```python
from build123d import *

# Parameters (mm, degrees)
SKETCH_1_W      = 54
SKETCH_1_H      = 35
EXTRUDE_1_DEPTH = 1.5
SKETCH_2_W      = 9.016092248
SKETCH_2_H      = 35
SKETCH_2_W_2    = 19.66831863
SKETCH_2_H_2    = 16.230096049
SKETCH_2_W_3    = 19.52262738
SKETCH_2_H_3    = 17.31299146
EXTRUDE_2_DEPTH = 9
SKETCH_3_W      = 19.66831863
SKETCH_3_H      = 16.230096049
SKETCH_3_W_2    = 19.52262738
SKETCH_3_H_2    = 17.31299146
EXTRUDE_3_DEPTH = 6


with BuildPart() as part:
    # 草图1 → 凸台-拉伸1 (new body)
    with BuildSketch(Plane(origin=(0, 0, 0), x_dir=(1, 0, 0), z_dir=(0, 1, 0))):
        with Locations((27, 119.607926306)):
            Rectangle(SKETCH_1_W, SKETCH_1_H)
    extrude(amount=EXTRUDE_1_DEPTH)

    # 草图2 → 凸台-拉伸2 (add)
    with BuildSketch(Plane(origin=(0, 1.5, 0), x_dir=(1, 0, 0), z_dir=(0, 1, 0))):
        with Locations((49.491953876, 119.607926306)):
            Rectangle(SKETCH_2_W, SKETCH_2_H)
        with Locations((33.692835946, 128.992878281)):
            Rectangle(SKETCH_2_W_2, SKETCH_2_H_2)
        with Locations((33.765681571, 110.764422036)):
            Rectangle(SKETCH_2_W_3, SKETCH_2_H_3)
    extrude(amount=EXTRUDE_2_DEPTH)

    # 草图3 → 凸台-拉伸3 (add)
    with BuildSketch(Plane(origin=(0, 10.5, 0), x_dir=(1, 0, 0), z_dir=(0, 1, 0))):
        with Locations((33.692835946, 128.992878281)):
            Rectangle(SKETCH_3_W, SKETCH_3_H)
        with Locations((33.765681571, 110.764422036)):
            Rectangle(SKETCH_3_W_2, SKETCH_3_H_2)
    extrude(amount=EXTRUDE_3_DEPTH)


solid = part.part
```
CAD build for the part. Positions are in the model's coordinates, mm. A direction names the side the tool comes from. Round coordinates to 2 decimals unless told otherwise and drop trailing zeros. Order: outer loops, then holes, each group sorted by start corner. A loop starts at its lowest first (then second) coordinate and runs counter-clockwise, first axis right, second up.
Q1. Drop flat-ended pins along their axis: pin 1 (12 mm diameter, centred on x = 12, z = -121, fed in from +Y); pin 2 (7.5 mm diameter, centred on y = 10, z = -107, fed in from -X); pin 3 (1.5 mm diameter, centred on x = 21, y = 4, fed in from +Z); pin 4 (7.5 mm diameter, centred on y = 8, z = -130, fed in from -X). Give the stop position or say it passes through.
Q2. Which spindle directions (+Z, -Z, +X, -X, +Y, -Y) get a long thin tool onto all of the face, cutting with end or side? Do faces 1 (the flat face through (23.859, 9, -129)), 2 (the flat face through (49, 10.5, -120)), 3 (the flat face through (43.527, 9, -129)), 4 (the flat face through (34, 9, -120.878)). Say none if no direction does.
Q3. Two-plate mould, pull along X, no slides. Class faces 5 (the flat face through (24.004, 9, -111)), 6 (the flat face through (43.527, 9, -111)), 7 (the flat face through (34, 16.5, -129)), 8 (the flat face through (54, 5, -119)): pulls with the +X half, pulls with the -X half, needs draft (parallel to the pull), parting line crosses it, or undercut.
Q4. Wall check: L1, parallel to Z at x = 24.5, y = 14.25; L2, parallel to X at y = 9, z = -131.5; L3, parallel to X at y = 9.5, z = -118. Give the ranges that are in metal, low to high.
Q5. Slice it at B-B (y = 4.25). Write the cut outline in (x, z).
Q6. Slice it at A-A (y = 14.75). Write the cut outline in (x, z), and give its area (3 significant figures).
Q7. Slice it at D-D (x = 27). Write the cut outline in (y, z), and give its area (3 significant figures).
Q8. Slice it at C-C (z = -113). Write the cut outline in (x, y), and give its area (3 significant figures).
Results below:
1. pin 1: stops at y = 1.5
1. pin 2: stops at x = 24
1. pin 3: passes through
1. pin 4: stops at x = 23.86
2. face 1: +Z, -Z, -X, +Y
2. face 2: +Z, -Z, +X, +Y
2. face 3: +Z, -Z, +Y
2. face 4: -X, +Y
3. face 5: pulls with the -X half
3. face 6: undercut
3. face 7: needs draft
3. face 8: pulls with the +X half
4. L1: z = -137.11 to -120.88, -119.42 to -102.11
4. L2: x = 23.86 to 43.53, 44.98 to 54
4. L3: x = 24 to 43.53, 44.98 to 54
5. outline: (23.86, -137.11) - (43.53, -137.11) - (43.53, -120.88) - (23.86, -120.88) - close; (24, -119.42) - (43.53, -119.42) - (43.53, -102.11) - (24, -102.11) - close; (44.98, -137.11) - (54, -137.11) - (54, -102.11) - (44.98, -102.11) - close
6. outline: (23.86, -137.11) - (43.53, -137.11) - (43.53, -120.88) - (23.86, -120.88) - close; (24, -119.42) - (43.53, -119.42) - (43.53, -102.11) - (24, -102.11) - close
6. area: 657 mm2
7. outline: (0, -137.11) - (16.5, -137.11) - (16.5, -120.88) - (1.5, -120.88) - (1.5, -119.42) - (16.5, -119.42) - (16.5, -102.11) - (0, -102.11) - close
7. area: 556 mm2
8. outline: (0, 0) - (54, 0) - (54, 10.5) - (44.98, 10.5) - (44.98, 1.5) - (43.53, 1.5) - (43.53, 16.5) - (24, 16.5) - (24, 1.5) - (0, 1.5) - close
8. area: 455 mm2
